from build123d import *

# Parameters (mm, degrees)
F0_R      = 19
F1_DEPTH  = 473
F2_R      = 16
F3_DEPTH  = 473.001
F4_R      = 16.175
F5_DEPTH  = 35
F6_R      = 16.175
F7_DEPTH  = 35
F10_D     = 5.5
F10_DEPTH = 20
F10_TIP   = 1.6523667023
F13_D     = 5
F13_DEPTH = 15
F13_TIP   = 1.5021515476


with BuildPart() as f1:
    # F0 (on Front) → F1 (new body)
    with BuildSketch(Plane.XZ):
        Circle(F0_R)
    extrude(amount=-F1_DEPTH)

    # F2 (on face) → F3 (cut, through all)
    with BuildSketch(Plane.XZ):
        Circle(F2_R)
    extrude(amount=-F3_DEPTH, mode=Mode.SUBTRACT)

    # F4 (on face) → F5 (cut)
    with BuildSketch(Plane.XZ):
        Circle(F4_R)
    extrude(amount=-F5_DEPTH, mode=Mode.SUBTRACT)

    # F6 (on face) → F7 (cut)
    with BuildSketch(Plane(origin=(0, 473, 0), x_dir=(-1, 0, 0), z_dir=(0, 1, 0))):
        Circle(F6_R)
    extrude(amount=-F7_DEPTH, mode=Mode.SUBTRACT)

    # F10
    with Locations(Plane.XY.offset(25)):
        with Locations((0, 96.5), (0, 111.5)):
            Hole(F10_D / 2, depth=F10_DEPTH)
            with Locations((0, 0, -(F10_DEPTH + F10_TIP / 2))):  # 118° drill point
                Cone(0, F10_D / 2, F10_TIP, mode=Mode.SUBTRACT)

    # F13
    with Locations(Plane(origin=(-25, 0, 0), x_dir=(0, 1, 0), z_dir=(-1, 0, 0))):
        with Locations((50, 0), (423, 0)):
            Hole(F13_D / 2, depth=F13_DEPTH)
            with Locations((0, 0, -(F13_DEPTH + F13_TIP / 2))):  # 118° drill point
                Cone(0, F13_D / 2, F13_TIP, mode=Mode.SUBTRACT)


solid = f1.part
Read the model definition and answer for the solid it produces. Units are mm, in the model's axes. Give positions to 0.01 mm unless a question says otherwise; leave off trailing zeros. Loops run counter-clockwise (first coordinate to the right, second up) from the corner with the lowest first, then second, coordinate; pieces in that order, holes last. Notation, with made-up numbers: M 38.5,25.5 L 58.5,25.5 A8 ccw 58.5,35.5 Z; hole C -28,-12 d8. An arc over 180 degrees is marked long. Write each question's results on one line, items separated by ' | '.
1. Straight lines are drawn through the part: line 1 (Y direction, x = 0, z = 17.1); line 2 (Z direction, x = 1, y = 186.5); line 3 (Z direction, x = -8.5, y = 382.5). For each, find the intervals that lie inside material, in ascending order. Write a range as [from, to].
Values:
line 1: y = [0, 93.75], [99.25, 108.75], [114.25, 473] | line 2: z = [-18.97, -15.97], [15.97, 18.97] | line 3: z = [-16.99, -13.56], [13.56, 16.99]
2. Section B-B on y = 76 is taken. Give the vertices of the cut face in (x, z), plus the area to 3 significant figures.
Values:
outline: C 0,0 d38; hole C 0,0 d32 | area: 330 mm^2
3. Given pin 1 (8 mm diameter, centred on y = 48, z = -15, fed in from +X); pin 2 (3 mm diameter, centred on x = -12, y = 50.5, fed in from +Z); pin 3 (6 mm diameter, centred on x = -10, y = 389.5, fed in from -Z), each flat-ended and moving along its own axis, determine where each tip first touches the part or whether it passes through.
Values:
pin 1: stops at x = 15.49 | pin 2: stops at z = 15.84 | pin 3: stops at z = -17.66
4. Section A-A on x = -10.5 is taken. Give the vertices of the cut face in (y, z), plus the area to 3 significant figures.
Values:
outline: M 0,-15.84 L 473,-15.84 L 473,-12.3 L 438,-12.3 L 438,-12.07 L 35,-12.07 L 35,-12.3 L 0,-12.3 Z; M 0,12.3 L 35,12.3 L 35,12.07 L 438,12.07 L 438,12.3 L 473,12.3 L 473,15.84 L 0,15.84 Z | area: 3,530 mm^2
5. The mould has two halves that part along X. Classify faces 1 (the face through (14, 0, 9)), 2 (the face through (-15.428, 455.745, 4.859)), 3 (the face through (8.767, 233.189, -16.856)): pulls with the +X half, pulls with the -X half, needs draft (parallel to the pull), parting line crosses it, or undercut.
Values:
face 1: needs draft | face 2: undercut | face 3: parting line crosses it
